The model under review builds one solid part; all positions refer to its coordinate system, in mm. Face numbers are marked on the shaded views. A direction names the side the tool comes from. Give positions to 0.01 mm unless a question says otherwise; leave off trailing zeros. Write each loop counter-clockwise with the first axis right and the second up, starting at its lowest first coordinate (ties: lowest second). Pieces come first, ordered by that corner, then holes. Notation, with made-up numbers: (87, -20.75) - (111, -20.75) arc R10 cw to (111, -14.75) - close; hole circle Ø3 at (38, 86.25). An arc over 180 degrees is marked (long way). Write item = value, one per line.
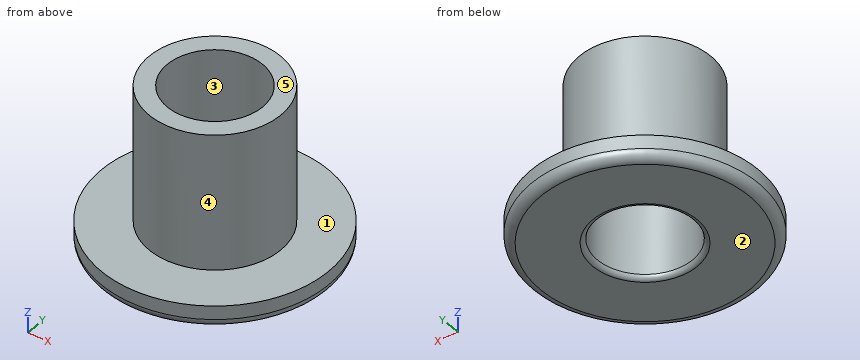
```python
from build123d import *

# Parameters (mm, degrees)
SKETCH1_R               = 5
BOSS_EXTRUDE1_DEPTH     = 1
SKETCH2_R               = 2.9
BOSS_EXTRUDE2_DEPTH     = 6
CUT_EXTRUDE2_DEPTH      = 10.949874371
CUT_EXTRUDE2_DEPTH_BACK = 10.949874371
SKETCH3_R               = 2.1
FILLET1_R               = 0.4
FILLET2_R               = 0.2


with BuildPart() as part:
    # Sketch1 → Boss-Extrude1 (new body)
    with BuildSketch(Plane.XY):
        Circle(SKETCH1_R)
    extrude(amount=BOSS_EXTRUDE1_DEPTH)

    # Sketch2 → Boss-Extrude2 (add)
    with BuildSketch(Plane.XY.offset(1)):
        Circle(SKETCH2_R)
    extrude(amount=BOSS_EXTRUDE2_DEPTH)

    # Sketch3 → Cut-Extrude2 (cut, two sides: drawn at the far end of the back side and taken through both)
    with BuildSketch(Plane.XY.offset(7).offset(-CUT_EXTRUDE2_DEPTH_BACK)):
        Circle(SKETCH3_R)
    extrude(amount=CUT_EXTRUDE2_DEPTH + CUT_EXTRUDE2_DEPTH_BACK, mode=Mode.SUBTRACT)

    # Fillet1
    fillet1_edges = [part.edges().sort_by_distance(p)[0] for p in [
        (-5, 0, 0),
    ]]
    fillet(fillet1_edges, radius=FILLET1_R)

    # Fillet2
    fillet2_edges = [part.edges().sort_by_distance(p)[0] for p in [
        (-2.1, 0, 0),
    ]]
    fillet(fillet2_edges, radius=FILLET2_R)


solid = part.part
```
1. Draft analysis for pull direction Y (two halves, no side actions). For the marked faces 3, 4 and 5, state which applies: +Y half, -Y half, draft (parallel to the pull), parting line (faces both ways), or undercut.
Findings below:
face_3 = undercut
face_4 = parting line
face_5 = draft
2. Insertion check: P1, Ø2, axis at x = 3, y = -1, coming from the +Z side; P2, Ø4, axis at y = -1.5, z = 4, coming from the +X side; P3, Ø1, axis at x = 1.5, y = -3.5, coming from the +Z side. Each pin has a flat end and moves straight along its axis. Give the tip position at first contact, or say it passes through.
Findings below:
P1 = 7
P2 = 2.9
P3 = 1
3. Machinability: for the marked faces 1 and 2, which of the approach directions +Z, -Z, +X, -X, +Y, -Y give a long, thin tool a straight path to every point of the face, cutting with its end or side? Answer none if there is none.
Findings below:
face_1 = +Z
face_2 = -Z, +X, -X, +Y, -Y
4. For line 1 (Y direction, x = 0, z = 3); line 2 (Z direction, x = 1.75, y = 4); line 3 (Y direction, x = 1.5, z = 4.5), list the stretches that pass through material, from the lowest coordinate up. Write a range as from..to.
Findings below:
line_1 = -2.9..-2.1, 2.1..2.9
line_2 = 0..1
line_3 = -2.48..-1.47, 1.47..2.48
5. Take a section at A-A on y = 0. Give the boundary of the cut face in (x, z), and give its area (3 significant figures).
Findings below:
outline = (-5, 0.4) arc R0.4 ccw to (-4.6, 0) - (-2.3, 0) arc R0.2 ccw to (-2.1, 0.2) - (-2.1, 7) - (-2.9, 7) - (-2.9, 1) - (-5, 1) - close; (2.1, 0.2) arc R0.2 ccw to (2.3, 0) - (4.6, 0) arc R0.4 ccw to (5, 0.4) - (5, 1) - (2.9, 1) - (2.9, 7) - (2.1, 7) - close
area = 15.3 mm²
